from build123d import *

# Parameters (mm, degrees)
F1_DEPTH = 600


with BuildPart() as f1:
    # F0 (on Front) → F1 (new body)
    with BuildSketch(Plane.XZ):
        with BuildLine():
            Line((5.400592, -15.418472), (3.027247, -7.405118))
            ThreePointArc((3.027247, -7.405118), (0, 8), (-3.027247, -7.405118))
            Line((-3.027247, -7.405118), (-5.400592, -15.418472))
            Line((-5.400592, -15.418472), (-5.400592, -20.151161))
            Line((-5.400592, -20.151161), (-20.206842, -20))
            Line((-20.206842, -20), (-20.206842, -25))
            Line((-20.206842, -25), (0, -25))
            Line((0, -25), (20.2184, -25))
            Line((20.2184, -25), (20.2184, -19.999882))
            Line((20.2184, -19.999882), (5.400592, -20.151161))
            Line((5.400592, -20.151161), (5.400592, -15.418472))
        make_face()
    extrude(amount=F1_DEPTH)


solid = f1.part
Can you work these out from the model? Positions are in its coordinate system, mm. Coordinates: 2 decimals unless noted, no trailing zeros. Write each loop counter-clockwise with the first axis right and the second up, starting at its lowest first coordinate (ties: lowest second). Pieces come first, ordered by that corner, then holes.
Q1. Please list where these lines run through material, in increasing order: L1, parallel to Z at x = 14.5, y = -256; L2, parallel to X at y = -224, z = -16.5; L3, parallel to Z at x = 7, y = -171.5.
Results found:
L1: z = -25 to -20.06
L2: x = -5.4 to 5.4
L3: z = -25 to -20.13, -3.87 to 3.87
Q2. Imagine slicing it at A-A, the plane y = -465. List the corners of the cut face in (x, z) for me, plus the area to 3 significant figures.
Results found:
outline: (-20.21, -25) - (20.22, -25) - (20.22, -20) - (5.4, -20.15) - (5.4, -15.42) - (3.03, -7.41) arc R8 ccw (long way) to (-3.03, -7.41) - (-5.4, -15.42) - (-5.4, -20.15) - (-20.21, -20) - close
area: 516 mm2
Q3. If we mould it in two halves opening along Z, with no side actions, what happens to faces 1 (the face through (0, -600, -12)), 2 (the face through (0, -296, -25)), 3 (the face through (0, -296, 8))? For each: +Z half, -Z half, draft (parallel to the pull), parting line (faces both ways), or undercut.
Results found:
face 1: draft
face 2: -Z half
face 3: undercut
Q4. For P1, Ø2, axis at x = 10.5, y = -86, coming from the +Z side; P2, Ø2, axis at y = -108.5, z = -3, coming from the -X side; P3, Ø8, axis at y = -400, z = 0, coming from the -X side; P4, Ø1.5, axis at x = -14.5, z = -20, coming from the +Y side, each with a flat end and sliding along its axis, tell me the tip position at first contact or that it passes through.
Results found:
P1: stops at z = -20.09
P2: stops at x = -7.75
P3: stops at x = -8
P4: stops at y = 0
Q5. Imagine slicing it at B-B, the plane z = 0. List the corners of the cut face in (x, y) for me.
Results found:
outline: (-8, -600) - (8, -600) - (8, 0) - (-8, 0) - close
